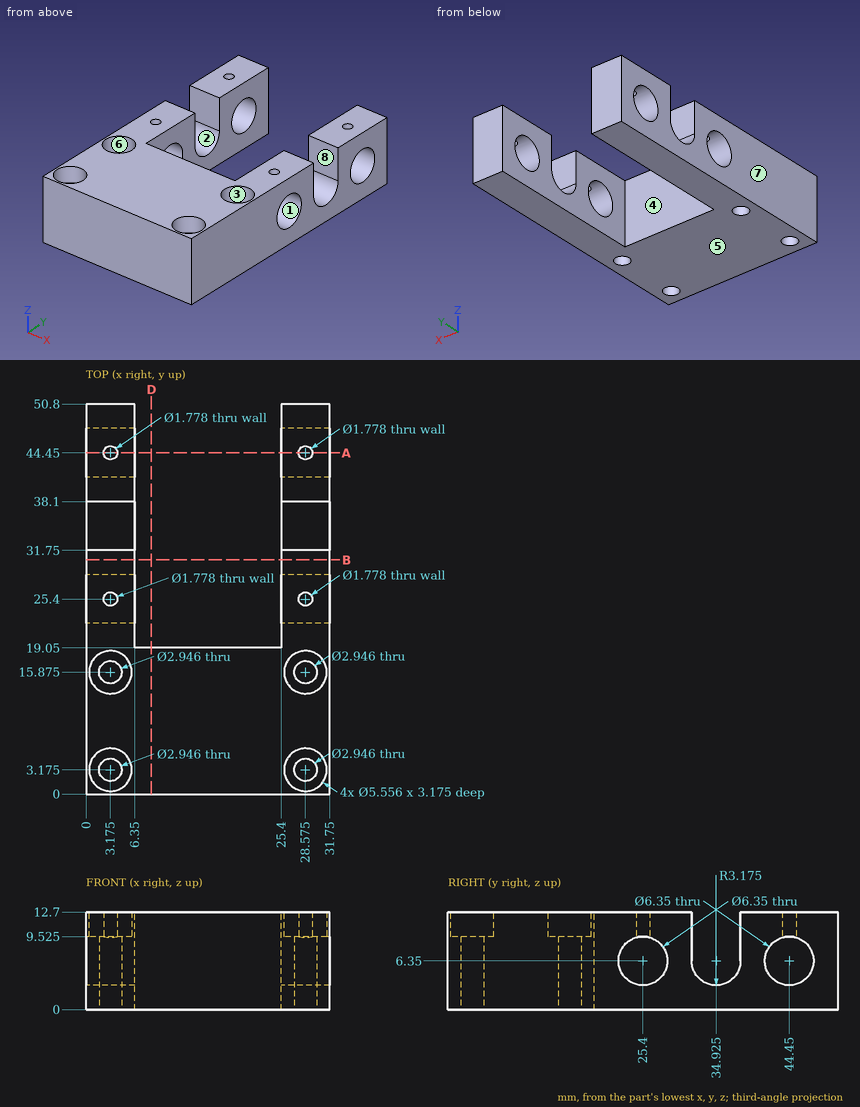
Study the drawing (mm; zero at the part's minimum x, y, z) and answer. A direction names the side the tool comes from. Round coordinates to 2 decimals unless told otherwise and drop trailing zeros. Write each loop counter-clockwise with the first axis right and the second up, starting at its lowest first coordinate (ties: lowest second). Pieces come first, ordered by that corner, then holes.
Q1. Straight lines are drawn through the part: line 1 (X direction, y = 26, z = 1.5); line 2 (Y direction, x = 2.5, z = 5.25) (1 decimal); line 3 (Y direction, x = 13, z = 9.25). For each, find the intervals that lie inside material, in ascending order.
Values:
line 1: x = 0 to 6.35, 25.4 to 31.75
line 2: y = 0 to 1.9, 4.5 to 14.6, 17.2 to 22.4, 28.4 to 31.9, 37.9 to 41.5, 47.4 to 50.8
line 3: y = 0 to 19.05
Q2. Find section A-A on y = 44.45. State how many separate pieces and enclosed holes the cut face has.
Values:
separate pieces: 6
enclosed holes: 0
Q3. Flat-ended cylindrical pins translate along their axes: P1, Ø4, axis at x = 21.5, y = 38.5, coming from the +Z side; P2, Ø3, axis at x = 11.5, z = 3.5, coming from the +Y side. Find the tip coordinate at first contact, or state that the pin passes through.
Values:
P1: passes through
P2: stops at y = 19.05
Q4. The mould has two halves that part along Z. Classify the marked faces 1, 2 and 3: released by +Z, released by -Z, zero draft, split by the parting line, or undercut.
Values:
face 1: undercut
face 2: released by +Z
face 3: zero draft
Q5. A tool of negligible diameter and unlimited length cuts with its end or side. For the marked faces 4, 5, 6, 7 and 8, from which of +Z, -Z, +X, -X, +Y, -Y can it reach the whole face along a straight path? Write none if from no direction.
Values:
face 4: +Z, -Z, +Y
face 5: -Z, +X, -X, +Y, -Y
face 6: +Z
face 7: +Z, -Z, -X, +Y, -Y
face 8: +Z, +X, -X
Q6. Find section D-D on x = 8.5. Determine the outline of the cut face in (y, z).
Values:
outline: (0, 0) - (19.05, 0) - (19.05, 12.7) - (0, 12.7) - close
Q7. Find section B-B on y = 30.5. Determine the outline of the cut face in (x, z), and give its area (3 significant figures).
Values:
outline: (0, 0) - (6.35, 0) - (6.35, 12.7) - (0, 12.7) - close; (25.4, 0) - (31.75, 0) - (31.75, 12.7) - (25.4, 12.7) - close
area: 161 mm2
